For this review, take the finished solid that the model builds, in its own axes (mm). A direction names the side the tool comes from. Give positions to 0.01 mm unless a question says otherwise; leave off trailing zeros. Write each loop counter-clockwise with the first axis right and the second up, starting at its lowest first coordinate (ties: lowest second). Pieces come first, ordered by that corner, then holes.
Q1. Insertion check: P1, Ø1.8, axis at x = 16.875, y = 73.5, coming from the +Z side; P2, Ø0.9, axis at x = -4, z = 1.5, coming from the +Y side; P3, Ø0.9, axis at x = 5, z = 1.5, coming from the -Y side. Each pin has a flat end and moves straight along its axis. Give the tip position at first contact, or say it passes through.
Q2. We need section D-D (y = 73.5). Write out the cut boundary in (x, z) (3 decimals), then the cut area to 4 significant figures.
Q3. We need section C-C (x = -3). Write out the cut boundary in (y, z).
Q4. Mouldability with a two-part tool opening along Y and no side actions: class faces 1 (the flat face through (5, 0, 1)), 2 (the flat face through (0, 56, 1)), 3 (the flat face through (17, 76, 2)), 4 (the cylindrical face through (-3, 34, 2)) as released by +Y, released by -Y, zero draft, split by the parting line, or undercut.
Q5. We need section B-B (z = 2.3). Write out the cut boundary in (x, y) (3 decimals).
Q6. For line 1 (Y direction, x = 21.5, z = 1.3); line 2 (Y direction, x = 17, z = 1.4); line 3 (X direction, y = 64.5, z = 1.35), list the stretches that pass through material, from the lowest coordinate up.
Q7. Machinability: for faces 5 (the flat face through (-3, 30.5, 2)), 6 (the flat face through (9.25, 73, 2)), 7 (the flat face through (-6, 35, 2)), which of the approach directions +Z, -Z, +X, -X, +Y, -Y give a long, thin tool a straight path to every point of the face, cutting with its end or side? Answer none if there is none.
Q8. We need section A-A (y = 35.5). Write out the cut boundary in (x, z).
Autodesk Inventor part; units mm, degrees
ref_plane "YZ Plane" through (0, 0, 0) normal (1, 0, 0) x (0, 1, 0)
ref_plane "XZ Plane" through (0, 0, 0) normal (0, 1, 0) x (-1, 0, 0)
ref_plane "XY Plane" through (0, 0, 0) normal (0, 0, 1) x (1, 0, 0)
sketch "Sketch1" plane through (0, 0, 0) normal (0, 0, 1) x (1, 0, 0)
  line L0 (0, 0) -> (18.5, 0)
  line L1 (0, 0) -> (0, 71)
  line L2 (0, 71) -> (18.5, 71)
  line L3 (18.5, 71) -> (18.5, 0)
  dimension "d0" = 18.5
  dimension "d1" = 71
extrude "Extrusion1" add sketch "Sketch1" along normal blind 3
sketch "Sketch2" plane through (0, 0, 3) normal (0, 0, 1) x (1, 0, 0)
  line L0 (0, 0) -> (18.5, 0)
  line L1 (18.5, 0) -> (18.5, 71)
  line L2 (18.5, 71) -> (0, 71)
  line L3 (0, 71) -> (0, 0)
  line L4 (24.5, 71) -> (24.5, 0)
  circle A0 centre (21.5, 64.5) radius 1.5
  circle A1 centre (21.5, 35.5) radius 1.5
  circle A2 centre (21.5, 6.5) radius 1.5
  line L5 (18.5, 71) -> (0, 71)
  line L6 (9.25, 71) -> (9.25, 76)
  line L7 (9.25, 76) -> (24.5, 76)
  line L8 (24.5, 76) -> (24.5, 71)
  circle A3 centre (16.875, 73.5) radius 1.5
  line L9 (0, 71) -> (0, 0)
  line L10 (9.25, 0) -> (9.25, -5)
  line L11 (9.25, -5) -> (24.5, -5)
  circle A4 centre (16.875, -2.5) radius 1.5
  line L12 (24.5, 0) -> (24.5, -5)
  dimension "d4" = 6
  dimension "d11" = 3
  dimension "d12" = 3
  dimension "d13" = 3
  dimension "d15" = 5
extrude "Extrusion2" add sketch "Sketch2" against normal blind 3 contours L0 L1 L2 L6 L7 L8 L4 L12 L11 L10
sketch "Sketch3" plane through (0, 0, 3) normal (0, 0, 1) x (1, 0, 0)
  line L0 (0, 71) -> (0, 0)
  line L1 (0, 35.5) -> (-6, 35.5)
  line L2 (-6, 35.5) -> (-6, 30.5)
  line L3 (-6, 30.5) -> (0, 30.5)
  line L4 (-6, 35.5) -> (-6, 40.5)
  line L5 (-6, 40.5) -> (0, 40.5)
  circle A0 centre (-3, 35.5) radius 1.5
  dimension "d19" = 6
  dimension "d20" = 5
  dimension "d21" = 5
  dimension "d22" = 3
extrude "Extrusion3" add sketch "Sketch3" against normal blind 3 contours L0 L1 A0 L4 L5 | L0 L3 L2 L1 A0
properties part number "side steel plates"
Computed:
1. P1: passes through
1. P2: stops at y = 40.5
1. P3: stops at y = 0
2. outline: (9.25, 0) - (15.375, 0) - (15.375, 3) - (9.25, 3) - close; (18.375, 0) - (24.5, 0) - (24.5, 3) - (18.375, 3) - close
2. area: 36.75 mm2
3. outline: (30.5, 0) - (34, 0) - (34, 3) - (30.5, 3) - close; (37, 0) - (40.5, 0) - (40.5, 3) - (37, 3) - close
4. face 1: released by -Y
4. face 2: zero draft
4. face 3: released by +Y
4. face 4: undercut
5. outline: (-6, 30.5) - (0, 30.5) - (0, 0) - (9.25, 0) - (9.25, -5) - (24.5, -5) - (24.5, 76) - (9.25, 76) - (9.25, 71) - (0, 71) - (0, 40.5) - (-6, 40.5) - close; hole circle Ø3 at (-3, 35.5); hole circle Ø3 at (16.875, -2.5); hole circle Ø3 at (16.875, 73.5); hole circle Ø3 at (21.5, 6.5); hole circle Ø3 at (21.5, 35.5); hole circle Ø3 at (21.5, 64.5)
6. line 1: y = -5 to 5, 8 to 34, 37 to 63, 66 to 76
6. line 2: y = -5 to -3.99, -1.01 to 72.01, 74.99 to 76
6. line 3: x = 0 to 20, 23 to 24.5
7. face 5: +Z, -Z, -X, -Y
7. face 6: +Z, -Z, -X, +Y
7. face 7: +Z, -Z, -X, +Y, -Y
8. outline: (-6, 0) - (-4.5, 0) - (-4.5, 3) - (-6, 3) - close; (-1.5, 0) - (20, 0) - (20, 3) - (-1.5, 3) - close; (23, 0) - (24.5, 0) - (24.5, 3) - (23, 3) - close
